The drawing under review shows one solid part. Ordinate dimensions are in mm from its lowest x, y, z. Round coordinates to 2 decimals unless told otherwise and drop trailing zeros. Order: outer loops, then holes, each group sorted by start corner. A loop starts at its lowest first (then second) coordinate and runs counter-clockwise, first axis right, second up. Notation, with made-up numbers: (89.5, -22) -> (96.5, -22) arc R25 ccw to (96.5, 7) -> close; hole circle Ø7 at (35.25, 64.5). An arc over 180 degrees is marked (long way). Use a Markdown table: item, result. Add a question column.
1) Draft analysis for pull direction X (two halves, no side actions). For the marked faces 1, 2 and 3, state which applies: pulls with the +X half, pulls with the -X half, needs draft (parallel to the pull), parting line crosses it, or undercut.
2) Clearance check with flat-ended pins moving along their axes: P1, Ø3, axis at y = 3.5, z = 19.5, coming from the +X side; P2, Ø4, axis at x = 4.5, z = 5.5, coming from the -Y side; P3, Ø3, axis at x = 7, y = 7, coming from the +Z side. State where each tip first meets the part, or that it passes through.
3) Consider section C-C (z = 20.75). State the section outline as (x, y) points.
4) Consider section A-A (z = 27.5). State the section outline as (x, y) points.
5) Consider section D-D (z = 6.25). State the section outline as (x, y) points, plus the area to 3 significant figures.
6) Wall thickness on line 1 along X through (y, z) = (7, 24.5); line 2 along X through (y, z) = (7, 23); line 3 along Y through (x, z) = (7, 25.5): over which ranges is each line inside the solid? List them lowest first. Write a range as [from, to].
7) Consider section B-B (z = 11.5). State the section outline as (x, y) points.
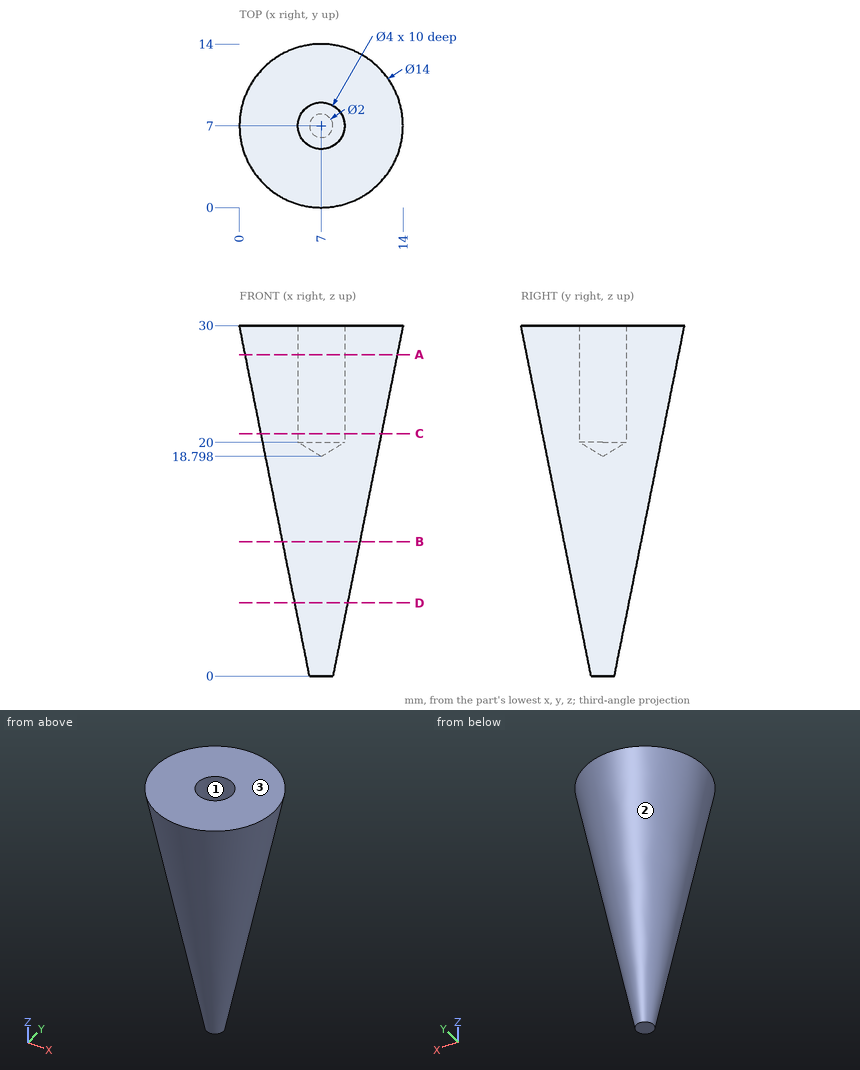
Results list:
| question | item | result |
|---|---|---|
| 1 | face 1 | undercut |
| 1 | face 2 | parting line crosses it |
| 1 | face 3 | needs draft |
| 2 | P1 | x = 11.55 |
| 2 | P2 | y = 4.83 |
| 2 | P3 | z = 19.7 |
| 3 | outline | circle Ø10.3 at (7, 7); hole circle Ø4 at (7, 7) |
| 4 | outline | circle Ø13 at (7, 7); hole circle Ø4 at (7, 7) |
| 5 | outline | circle Ø4.5 at (7, 7) |
| 5 | area | 15.9 mm2 |
| 6 | line 1 | [1.1, 5], [9, 12.9] |
| 6 | line 2 | [1.4, 5], [9, 12.6] |
| 6 | line 3 | [0.9, 5], [9, 13.1] |
| 7 | outline | circle Ø6.6 at (7, 7) |
